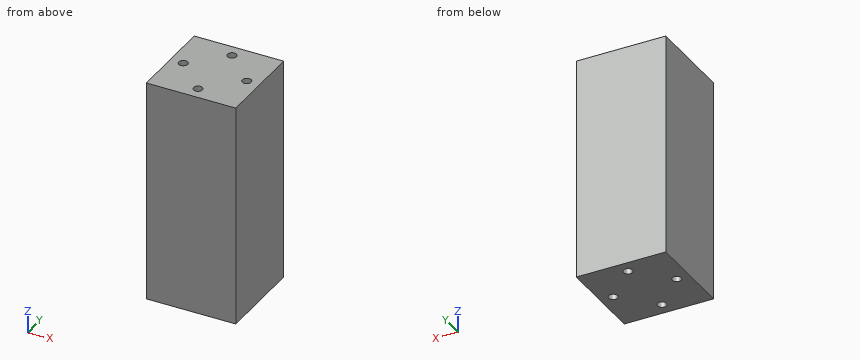
from build123d import *

# Parameters (mm, degrees)
SKETCH_1_W          = 20
SKETCH_1_H          = 20
EXTRUDE_1_DEPTH     = 50
SKETCH_1_3_R        = 1
CUT_EXTRUDE_1_DEPTH = 3
CUT_EXTRUDE_START   = 47
SKETCH_1_4_R        = 1
CUT_EXTRUDE_2_DEPTH = 3


with BuildPart() as part:
    # 草图1 → 凸台-拉伸1 (new body)
    with BuildSketch(Plane.XY):
        Rectangle(SKETCH_1_W, SKETCH_1_H)
    extrude(amount=EXTRUDE_1_DEPTH)

    # 草图1<3> → 切除-拉伸1 (cut)
    with BuildSketch(Plane.XY):
        with Locations((-7.1, 0)):
            Circle(SKETCH_1_3_R)
        with Locations((0, 7.1)):
            Circle(SKETCH_1_3_R)
        with Locations((7.1, 0)):
            Circle(SKETCH_1_3_R)
        with Locations((0, -7.1)):
            Circle(SKETCH_1_3_R)
    extrude(amount=CUT_EXTRUDE_1_DEPTH, mode=Mode.SUBTRACT)

    # 草图1<4> → 切除-拉伸2 (cut)
    with BuildSketch(Plane.XY.offset(CUT_EXTRUDE_START)):
        with Locations((-7.1, 0)):
            Circle(SKETCH_1_4_R)
        with Locations((0, 7.1)):
            Circle(SKETCH_1_4_R)
        with Locations((7.1, 0)):
            Circle(SKETCH_1_4_R)
        with Locations((0, -7.1)):
            Circle(SKETCH_1_4_R)
    extrude(amount=CUT_EXTRUDE_2_DEPTH, mode=Mode.SUBTRACT)


solid = part.part
Source: CAD feature listing. Evaluate the final solid. Frame: model axes, mm. Round coordinates to 2 decimals unless told otherwise and drop trailing zeros. Order: outer loops, then holes, each group sorted by start corner. A loop starts at its lowest first (then second) coordinate and runs counter-clockwise, first axis right, second up. Notation, with made-up numbers: (88.5, 10.25) -> (114.5, 10.25) arc R22 ccw to (114.5, 19.25) -> close; hole circle Ø3 at (58.5, -5.5). An arc over 180 degrees is marked (long way). Answer as CSV lines item,"result".
Item 1: Section A-A, the plane y = 0. Return loops of the section in (x, z).
A:
outline,"(-10, 0) -> (-8.1, 0) -> (-8.1, 3) -> (-6.1, 3) -> (-6.1, 0) -> (6.1, 0) -> (6.1, 3) -> (8.1, 3) -> (8.1, 0) -> (10, 0) -> (10, 50) -> (8.1, 50) -> (8.1, 47) -> (6.1, 47) -> (6.1, 50) -> (-6.1, 50) -> (-6.1, 47) -> (-8.1, 47) -> (-8.1, 50) -> (-10, 50) -> close"
Item 2: Line query: L1, parallel to Y at x = -7.1, z = 48.75. Output: solid intervals per line, ascending.
A:
L1,"-10 to -1, 1 to 10"
Item 3: Pin query (flat end, axial travel): pin 1 Ø1.2 at (x, y) = (-7.1, 0) entering from -Z; pin 2 Ø1.8 at (x, y) = (-7.1, 0) entering from +Z. Return the tip coordinate at first contact, or that it passes through.
A:
pin 1,"z = 3"
pin 2,"z = 47"
